```python
from build123d import *

# Parameters (mm, degrees)
F1_DEPTH = 4
F2_R     = 2
F3_R     = 5


with BuildPart() as f1:
    # F0 (on Top) → F1 (new body)
    with BuildSketch(Plane.XY):
        with BuildLine():
            Line((-30.803579, 38.437911), (-11.687509, 5.327906))
            Line((-11.687509, 5.327906), (-11.687509, 2.830331))
            ThreePointArc((-11.687509, 2.830331), (-11.199892, 2.342714), (-10.712276, 2.830331))
            Line((-10.712276, 2.830331), (-2.687509, 2.830331))
            Line((-2.687509, 2.830331), (-2.687509, -27.169669))
            Line((-2.687509, -27.169669), (-10.712276, -27.169669))
            ThreePointArc((-10.712276, -27.169669), (-11.199892, -26.682053), (-11.687509, -27.169669))
            Line((-11.687509, -27.169669), (-11.687509, -30.672094))
            Line((-11.687509, -30.672094), (0.312491, -30.672094))
            Line((0.312491, -30.672094), (6.158749, 5.327906))
            Line((6.158749, 5.327906), (-17.460834, 46.238223))
            Line((-17.460834, 46.238223), (-24.356114, 42.207168))
            Line((-24.356114, 42.207168), (-14.269803, 24.954133))
            Line((-14.269803, 24.954133), (-15.305761, 24.3485))
            Line((-15.305761, 24.3485), (-25.392072, 41.601536))
            Line((-25.392072, 41.601536), (-30.803579, 38.437911))
        make_face()
    extrude(amount=F1_DEPTH)

    # F2
    f2_edges = [f1.edges().sort_by_distance(p)[0] for p in [
        (0.312491, -30.672094, 2),
        (-11.687509, -30.672094, 2),
        (-17.460834, 46.238223, 2),
        (-30.803579, 38.437911, 2),
    ]]
    fillet(f2_edges, radius=F2_R)

    # F3
    f3_edges = [f1.edges().sort_by_distance(p)[0] for p in [
        (6.158749, 5.327906, 2),
        (-11.687509, 5.327906, 2),
    ]]
    fillet(f3_edges, radius=F3_R)


solid = f1.part
```
Can you work these out from the model? Positions are in its coordinate system, mm. A direction names the side the tool comes from. Give positions to 0.01 mm unless a question says otherwise; leave off trailing zeros. Order: outer loops, then holes, each group sorted by start corner. A loop starts at its lowest first (then second) coordinate and runs counter-clockwise, first axis right, second up. Notation, with made-up numbers: M 30,68 L 83,68 A23 cw 83,84 Z; hole C 34.25,38 d3. An arc over 180 degrees is marked long. Write item = value, one per line. Start each with the question number.
Q1. Suppose I cut it at B-B (z = 1.7). Write out the boundary of the cut face in (x, y), plus the area to 3 significant figures.
Q2. We'd pull the mould along X, two halves only. Please class faces 1 (the flat face through (-6, -30.672, 2)), 2 (the flat face through (-7, -27.17, 2)), 3 (the cylindrical face through (5.85, 5.3, 2.03)), 4 (the flat face through (-21.74, 43.736, 1.972)): pulls with the +X half, pulls with the -X half, needs draft (parallel to the pull), parting line crosses it, or undercut.
Q3. For faces 5 (the flat face through (-19.384, 33.701, 1.972)), 6 (the flat face through (-11, 16, 0)), 7 (the flat face through (-11.688, -28, 2)), which set-ups out of +Z, -Z, +X, -X, +Y, -Y let a thin tool reach every point of the face, with its end or its side?
Q4. Suppose I cut it at C-C (x = -7). Write out the boundary of the cut face in (y, z).
Q5. Suppose I cut it at A-A (x = -22.5). Write out the boundary of the cut face in (y, z), plus the area to 3 significant figures.
Q6. Will these pins go through, and if not, where does the flat tip stop? pin 1 Ø2 at (x, z) = (-6, 1.5) entering from +Y; pin 2 Ø0.8 at (y, z) = (-28, 1.5) entering from -X; pin 3 Ø1 at (x, z) = (-23.5, 1) entering from -Y.
Q7. Suppose I cut it at D-D (y = -9). Write out the boundary of the cut face in (x, z).
Q8. I need wall thicknesses on probe 1 along Y at (x, z) = (-9, 0.5); probe 2 along Y at (x, z) = (-16, 0.6); probe 3 along X at (y, z) = (40, 3.6). Which ranges of each line are inside material? Lowest first, please. Write a range as [from, to].
Check result:
q1.outline = M -29.81,36.72 L -12.36,6.49 A5 cw -11.69,3.99 L -11.69,2.83 A0.49 ccw -10.71,2.83 L -2.69,2.83 L -2.69,-27.17 L -10.71,-27.17 A0.49 ccw -11.69,-27.17 L -11.69,-28.67 A2 ccw -9.69,-30.67 L -1.39,-30.67 A2 ccw 0.59,-28.99 L 5.87,3.57 A5 ccw 5.27,6.87 L -16.46,44.5 A2 ccw -19.2,45.22 L -24.36,42.21 L -14.27,24.95 L -15.31,24.35 L -25.39,41.6 L -29.09,39.44 A2 ccw Z
q1.area = 901 mm2
q2.face_1 = needs draft
q2.face_2 = undercut
q2.face_3 = pulls with the +X half
q2.face_4 = pulls with the -X half
q3.face_5 = +Z, -Z
q3.face_6 = -Z, +X, -X, +Y, -Y
q3.face_7 = +Z, -Z, -X, -Y
q4.outline = M -30.67,0 L -27.17,0 L -27.17,4 L -30.67,4 Z; M 2.83,0 L 28.12,0 L 28.12,4 L 2.83,4 Z
q5.outline = M 24.06,0 L 36.65,0 L 36.65,4 L 24.06,4 Z; M 39.03,0 L 43.29,0 L 43.29,4 L 39.03,4 Z
q5.area = 67.4 mm2
q6.pin_1 = 28.12
q6.pin_2 = -11.69
q6.pin_3 = 24.92
q7.outline = M -2.69,0 L 3.83,0 L 3.83,4 L -2.69,4 Z
q8.probe_1 = [-30.67, -27.17], [2.83, 31.58]
q8.probe_2 = [12.8, 25.54], [27.91, 43.71]
q8.probe_3 = [-28.13, -24.46], [-23.07, -13.86]
